Read the model definition and answer for the solid it produces. Units are mm, in the model's axes. A direction names the side the tool comes from. Round coordinates to 2 decimals unless told otherwise and drop trailing zeros. Order: outer loops, then holes, each group sorted by start corner. A loop starts at its lowest first (then second) coordinate and runs counter-clockwise, first axis right, second up. Notation, with made-up numbers: (-5, -17) - (27, -17) arc R20 cw to (27, 0) - close; hole circle Ø8 at (35, -18.75). An arc over 180 degrees is marked (long way). One line per question, with ' | ' between items. Start each with the question number.
1) For faces 1 (the cylindrical face through (-47.1, -3.94, -39.14)), 2 (the flat face through (-26, 0, 1)), determine the directions among +Z, -Z, +X, -X, +Y, -Y from which every point of the face is accessible in a straight line to the end or side of a thin tool.
2) The part is cut by section C-C, the plane z = -0.5. Give the vertices of the cut face in (x, y).
3) The part is cut by section A-A, the plane x = -36. Give the vertices of the cut face in (y, z).
4) The mould has two halves that part along X. Classify faces 3 (the flat face through (0, 17, 1)), 4 (the flat face through (-12.5, -0.4, -40)), 5 (the cylindrical face through (4.863, -4.692, 0.56)), 6 (the cylindrical face through (-37.21, -3.94, 25.51)): pulls with the +X half, pulls with the -X half, needs draft (parallel to the pull), parting line crosses it, or undercut.
5) The part is cut by section D-D, the plane y = -5.5. Give the vertices of the cut face in (x, z).
6) Flat-ended cylindrical pins translate along their axes: pin 1 (2 mm diameter, centred on x = -8.5, z = 1, fed in from +Y); pin 2 (3 mm diameter, centred on y = 27.5, z = -13.5, fed in from -X). Find the tip coordinate at first contact, or state that the pin passes through.
7) Straight lines are drawn through the part: line 1 (Y direction, x = -26, z = 9.5); line 2 (X direction, y = 13, z = 8.5); line 3 (Y direction, x = 3, z = 0). For each, find the intervals that lie inside material, in ascending order. Write a range as from..to.
8) The part is cut by section B-B, the plane y = 24. Give the vertices of the cut face in (x, z), plus the area to 3 significant figures.
from build123d import *

# Parameters (mm, degrees)
BASE_FLANGE1_DEPTH = 40
FILLET1_R          = 3
SKETCH6_R          = 3.15
CUT_EXTRUDE1_DEPTH = 10
SKETCH7_R          = 3
CUT_EXTRUDE2_DEPTH = 10


# Sheet-metal steps are written as plain solids
with BuildPart() as part:
    # Sketch1 → Base-Flange1 (new, symmetric)
    with BuildSketch(Plane.XY):
        with BuildLine():
            Line((-48, 0), (-3, 0))
            ThreePointArc((-3, 0), (-0.878679656, 0.878679656), (0, 3))
            Line((0, 3), (0, 32))
            Line((0, 32), (8, 32))
            Line((8, 32), (8, 3))
            ThreePointArc((8, 3), (4.778174593, -4.778174593), (-3, -8))
            Line((-3, -8), (-48, -8))
            Line((-48, -8), (-48, 0))
        make_face()
    extrude(amount=BASE_FLANGE1_DEPTH, both=True)

    # Fillet1
    fillet1_edges = [part.edges().sort_by_distance(p)[0] for p in [
        (-48, -4, 40),
        (-48, -4, -40),
        (4, 32, 40),
        (4, 32, -40),
    ]]
    fillet(fillet1_edges, radius=FILLET1_R)

    # Sketch6 → Cut-Extrude1 (cut)
    with BuildSketch(Plane(origin=(0, 0, 0), x_dir=(1, 0, 0), z_dir=(0, 1, 0))):
        with Locations(Location((-36, 25.397681591, 0), (0, 0, 270))):
            Circle(SKETCH6_R)
        with Locations(Location((-36, -22.602318409, 0), (0, 0, 270))):
            Circle(SKETCH6_R)
    extrude(amount=-CUT_EXTRUDE1_DEPTH, mode=Mode.SUBTRACT)

    # Sketch7 → Cut-Extrude2 (cut)
    with BuildSketch(Plane.ZY):
        with Locations((0, 24)):
            Circle(SKETCH7_R)
    extrude(amount=-CUT_EXTRUDE2_DEPTH, mode=Mode.SUBTRACT)


solid = part.part
Values:
1) face 1: -Z, -X, +Y, -Y | face 2: +Z, -Z, -X, +Y
2) outline: (-48, -8) - (-3, -8) arc R11 ccw to (8, 3) - (8, 21.04) - (0, 21.04) - (0, 3) arc R3 cw to (-3, 0) - (-48, 0) - close; (0, 26.96) - (8, 26.96) - (8, 32) - (0, 32) - close
3) outline: (-8, -40) - (0, -40) - (0, -28.55) - (-8, -28.55) - close; (-8, -22.25) - (0, -22.25) - (0, 19.45) - (-8, 19.45) - close; (-8, 25.75) - (0, 25.75) - (0, 40) - (-8, 40) - close
4) face 3: pulls with the -X half | face 4: needs draft | face 5: pulls with the +X half | face 6: undercut
5) outline: (-48, -37) arc R3 ccw to (-45, -40) - (3.98, -40) - (3.98, 40) - (-45, 40) arc R3 ccw to (-48, 37) - close; hole circle Ø6.3 at (-36, -25.4); hole circle Ø6.3 at (-36, 22.6)
6) pin 1: stops at y = 0 | pin 2: stops at x = 0
7) line 1: y = -8..0 | line 2: x = 0..8 | line 3: y = -6.22..21, 27..32
8) outline: (0, -40) - (8, -40) - (8, -3) - (0, -3) - close; (0, 3) - (8, 3) - (8, 40) - (0, 40) - close | area: 592 mm^2
